Geometry: final body of the model. Coordinates: model frame, mm. Round coordinates to 2 decimals unless told otherwise and drop trailing zeros. Loops run counter-clockwise (first coordinate to the right, second up) from the corner with the lowest first, then second, coordinate; pieces in that order, holes last. Notation, with made-up numbers: (-1, 62) - (37, 62) arc R8 ccw to (37, 70) - close; hole circle Ø1 at (32, 19). An arc over 180 degrees is marked (long way). Answer as a JSON object with one key per item and string values. Group by question number.
Item 1: First-contact query: pin 1 (3 mm diameter, centred on x = -43.5, y = -84.5, fed in from -Z); pin 2 (2 mm diameter, centred on x = -61.5, y = -18.5, fed in from -Z); pin 3 (4 mm diameter, centred on x = -36.5, y = -19.5, fed in from +Z). Flat tips, straight axial feed; report the tip coordinate or a pass-through.
Item 2: Section A-A (y = -99.5). Return the cut outline in (x, z) (3 decimals).
Item 3: Line query: line 1 (Z direction, x = -52, y = -106.5); line 2 (Z direction, x = -50, y = -108.5); line 3 (X direction, y = -43, z = 31.5). Output: solid intervals per line, ascending.
Item 4: Section B-B (y = -120). Return the cut outline in (x, z).
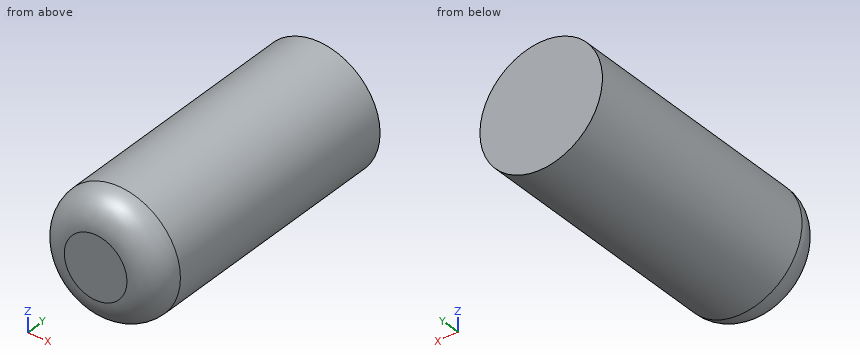
```python
from build123d import *

# Parameters (mm, degrees)
F0_R     = 28.575
F1_DEPTH = 132.37323
F2_R     = 20.952387
F3_DEPTH = 17.41577
F4_R     = 13.961373


with BuildPart() as f1:
    # F0 (on Front) → F1 (new body)
    with BuildSketch(Plane.XZ):
        with Locations((-50.799999, 25.400002)):
            Circle(F0_R)
    extrude(amount=F1_DEPTH)

    # F2 (on face) → F3 (join)
    with BuildSketch(Plane.XZ.offset(132.37323)):
        with Locations((-50.799999, 25.400002)):
            Circle(F2_R)
    extrude(amount=-F3_DEPTH)

    # F4
    f4_edges = [f1.edges().sort_by_distance(p)[0] for p in [
        (-79.374999, -132.37323, 25.400002),
    ]]
    fillet(f4_edges, radius=F4_R)


solid = f1.part
```
Values:
{
 "1": {"pin 1": "stops at z = -2.58", "pin 2": "stops at z = -1.48", "pin 3": "stops at z = 51.19"},
 "2": {"outline": "circle Ø57.15 at (-50.8, 25.4)"},
 "3": {"line 1": "z = -3.15 to 53.95", "line 2": "z = -3.16 to 53.96", "line 3": "x = -78.72 to -22.88"},
 "4": {"outline": "circle Ø56.97 at (-50.8, 25.4)"}
}
